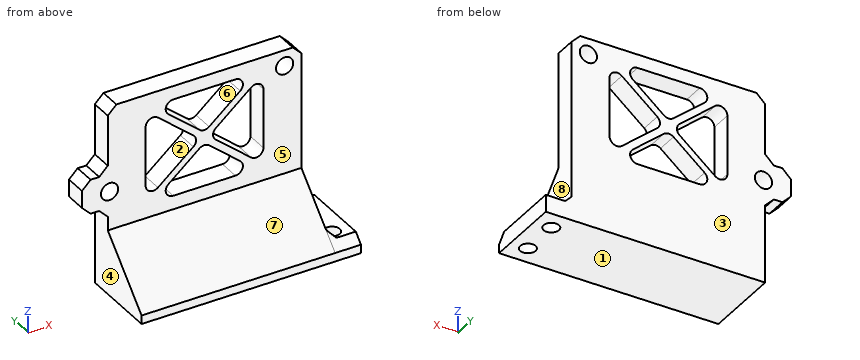
Autodesk Inventor part; units mm, degrees
ref_plane "作業平面2" through (-4, 15.3, 26.3) normal (0, -1, 0) x (1, 0, 0)
ref_plane "作業平面1" through (-4, 15.3, 26.3) normal (0, -1, 0) x (1, 0, 0)
ref_plane "作業平面3" through (45, 13, 3) normal (0, -1, 0) x (1, 0, 0)
sketch "スケッチ1" plane through (0, 0, 0) normal (0, 0, 1) x (1, 0, 0)
  line L0 (0, 0) -> (51, 0)
  line L1 (51, 0) -> (51, 18)
  line L2 (51, 18) -> (0, 18)
  line L3 (0, 18) -> (0, 0)
  circle A0 centre (47, 13.5) radius 1.8
  circle A1 centre (47, 4.5) radius 1.8
  dimension "d0" = 51
  dimension "d1" = 18
  dimension "d4" = 3.6
  dimension "d5" = 13.5
  dimension "d6" = 4
  dimension "d7" = 3.6
  dimension "d8" = 4
  dimension "d9" = 4.5
extrude "押し出し2" add sketch "スケッチ1" along normal blind 2
sketch "スケッチ2" plane through (0, 0, 2) normal (0, 0, 1) x (1, 0, 0)
  line L0 (0, 18) -> (0, 0)
  line L1 (0, 18) -> (44, 18)
  line L2 (44, 18) -> (44, 13)
  line L3 (44, 13) -> (0, 13)
  line L4 (0, 13) -> (0, 18)
  dimension "d12" = 44
  dimension "d13" = 5
extrude "押し出し3" add sketch "スケッチ2" along normal blind 42
sketch "スケッチ3" plane through (0, 13, 2) normal (0, -1, 0) x (1, 0, 0)
  circle A0 centre (41.1, 3.5) radius 2
  line L0 (44, 0) -> (44, 42)
  line L1 (44, 0) -> (0, 0)
  circle A1 centre (0.4, 19.8) radius 2
  point P0 (0, -2)
  dimension "d16" = 4
  dimension "d17" = 2.9
  dimension "d18" = 3.5
  dimension "d27" = 4
  dimension "d28" = 40.7
  dimension "d29" = 16.3
sketch "スケッチ4" plane through (0, 13, 2) normal (0, -1, 0) x (1, 0, 0)
  line L0 (8, 13.3) -> (-4, 13.3)
  line L1 (-4, 13.3) -> (-4, 24.3)
  line L2 (-4, 24.3) -> (8, 24.3)
  line L3 (8, 24.3) -> (8, 13.3)
  line L4 (44, 0) -> (0, 0)
  line L5 (44, 0) -> (44, 42)
  line L6 (0, 42) -> (44, 42)
  line L7 (0, 0) -> (0, 42)
  point P0 (0, -2)
  dimension "d19" = 13.3
  dimension "d20" = 36
  dimension "d25" = 11
  dimension "d26" = 12
ref_plane "作業平面2" through (-4, 15.3, 26.3) normal (0, -1, 0) x (1, 0, 0)
sketch "スケッチ5" plane through (-4, 15.3, 26.3) normal (0, -1, 0) x (1, 0, 0)
  point P0 (4, -26.3)
ref_plane "作業平面1" through (-4, 15.3, 26.3) normal (0, -1, 0) x (1, 0, 0)
sketch "スケッチ6" plane through (-4, 15.3, 26.3) normal (0, -1, 0) x (1, 0, 0)
  line L0 (4, -24.3) -> (4, 17.7)
  circle A0 centre (4.4, -2.3) radius 2
  circle A1 centre (45.1, 14) radius 2
  line L1 (4, -24.3) -> (55, -24.3)
  line L2 (48, -24.3) -> (48, 17.7)
  line L3 (4, 17.7) -> (48, 17.7)
  point P0 (4, -26.3)
  dimension "d45" = 4
  dimension "d46" = 0.4
  dimension "d47" = 4
  dimension "d48" = 22
  dimension "d49" = 2.9
  dimension "d67" = 43.8427
sketch "スケッチ7" plane through (0, 13, 2) normal (0, -1, 0) x (1, 0, 0)
  point P0 (0, -2)
sketch "スケッチ8" plane through (0, 13, 2) normal (0, -1, 0) x (1, 0, 0)
  line L0 (44, 0) -> (44, 42)
  line L1 (44, 0) -> (45, 0)
  line L2 (45, 0) -> (45, 21.3)
  line L3 (45, 21.3) -> (44, 21.3)
  line L4 (44, 21.3) -> (44, 0)
  point P0 (0, -2)
  dimension "d35" = 1
extrude "押し出し6" add sketch "スケッチ8" against normal blind 5
ref_plane "作業平面3" through (45, 13, 3) normal (0, -1, 0) x (1, 0, 0)
sketch "スケッチ9" plane through (45, 13, 3) normal (0, -1, 0) x (1, 0, 0)
  line L0 (-51, 17.2309) -> (-43, 17.2309)
  line L1 (-43, 17.2309) -> (-43, 25.2309)
  line L2 (-43, 25.2309) -> (-51, 25.2309)
  line L3 (-51, 25.2309) -> (-51, 17.2309)
  line L4 (0, 41) -> (-10, 41)
  line L5 (-10, 41) -> (-10, 7.258)
  line L6 (-10, 7.258) -> (0, 7.258)
  line L7 (0, 7.258) -> (0, 41)
  line L8 (0, 16.7) -> (0, 41)
  line L9 (-45, -1) -> (6, -1)
  point P0 (-45, -3)
  point P1 (-45, 4.4596)
  point P2 (-2.5771, 20.3)
  dimension "d55" = 8
  dimension "d59" = 0
  dimension "d97" = 18.2309
  dimension "d98" = 8.258
  dimension "d99" = 33.742
extrude "押し出し8" add sketch "スケッチ9" against normal blind 5
extrude "押し出し9" cut sketch "スケッチ6" along normal mid plane 10 contours A0 L0 | L0 A0 | A1
chamfer "面取り5" distance 13 angle 45 1 edges at (22.5, 13, 2)
sketch "スケッチ10" plane through (0, 0, 2) normal (0, 0, 1) x (1, 0, 0)
  line L0 (45, 18) -> (45, 0)
  line L1 (45, 0) -> (51, 0)
  line L2 (51, 0) -> (51, 18)
  line L3 (51, 18) -> (45, 18)
  circle A0 centre (47, 13.5) radius 1.8
  circle A1 centre (47, 4.5) radius 1.8
  circle A2 centre (47, 4.5) radius 1.8
  circle A3 centre (47, 13.5) radius 1.8
  line L4 (45, 0) -> (51, 0)
  line L5 (51, 0) -> (51, 18)
  line L6 (51, 18) -> (45, 18)
  line L7 (45, 18) -> (45, 0)
  point P0 (0, 0)
extrude "押し出し10" add sketch "スケッチ10" along normal blind 2
chamfer "面取り6" distance 2 angle 45 1 edges at (48, 0, 4)
chamfer "面取り7" distance 1.5 angle 45 1 edges at (45, 10.0001, 4)
chamfer "面取り8" distance 2 angle 45 4 edges at (45, 15.5, 44) (0, 15.5, 44) (-6, 15.5, 20.2309) (-6, 15.5, 28.2309)
sketch "スケッチ11" plane through (0, 13, 15) normal (0, -1, 0) x (1, 0, 0)
  line L0 (45, 0) -> (45, 27)
  line L1 (45, 13.5) -> (35.6998, 13.5)
  line L2 (19.8872, 15.8543) -> (11.6558, 22.7612)
  line L3 (21.4786, 14.5189) -> (32.2238, 14.5189) construction
  line L4 (19.8872, 13.1836) -> (11.6558, 6.2766)
  line L5 (21.4786, 14.5189) -> (32.2239, 14.5189) construction
  line L6 (8.7921, 7.612) -> (8.7921, 21.4259)
  arc A0 (11.6558, 22.7612) -> (8.7921, 21.4259) centre (10.5353, 21.4258) ccw
  arc A1 (19.8872, 13.1836) -> (19.8872, 15.8543) centre (18.7667, 14.5189) ccw
  arc A2 (8.7921, 7.612) -> (11.6558, 6.2766) centre (10.5353, 7.612) ccw
  line L7 (25.0769, 15.8544) -> (33.3082, 22.7613)
  line L8 (25.0769, 13.1835) -> (33.3082, 6.2766)
  line L9 (36.1721, 7.612) -> (36.1721, 21.4258)
  arc A3 (36.1721, 21.4258) -> (33.3082, 22.7613) centre (34.4288, 21.4258) ccw
  arc A4 (25.0769, 15.8544) -> (25.0769, 13.1835) centre (26.1975, 14.5189) ccw
  arc A5 (33.3082, 6.2766) -> (36.1721, 7.612) centre (34.4288, 7.612) ccw
  line L10 (23.55, 16.7078) -> (30.7794, 22.774)
  line L11 (23.8988, 16.5352) -> (33.3361, 16.5352) construction
  line L12 (21.3092, 16.7078) -> (14.0798, 22.774)
  line L13 (23.8988, 16.5352) -> (33.3361, 16.5352) construction
  line L14 (15.2002, 25.8522) -> (29.659, 25.8522)
  arc A6 (21.3092, 16.7078) -> (23.55, 16.7078) centre (22.4296, 18.043) ccw
  arc A7 (15.2002, 25.8522) -> (14.0798, 22.774) centre (15.2002, 24.1092) ccw
  arc A8 (30.7794, 22.774) -> (29.659, 25.8522) centre (29.659, 24.1092) ccw
  line L15 (23.5502, 12.3302) -> (30.7795, 6.2641)
  line L16 (21.309, 12.3302) -> (14.0797, 6.2641)
  line L17 (15.2003, 3.1853) -> (29.6589, 3.1853)
  arc A9 (23.5502, 12.3302) -> (21.309, 12.3302) centre (22.4296, 10.9947) ccw
  arc A10 (14.0797, 6.2641) -> (15.2003, 3.1853) centre (15.2003, 4.9286) ccw
  arc A11 (29.6589, 3.1853) -> (30.7795, 6.2641) centre (29.6589, 4.9286) ccw
  point P0 (0, -15)
  point P1 (8.7921, 25.1641)
  point P2 (8.792, 3.8737)
  point P3 (23.4854, 14.5189)
  point P4 (36.1721, 25.1643)
  point P5 (36.1721, 3.8735)
  point P6 (35.918, 26.6205)
  point P7 (11.8795, 26.6205)
  point P8 (21.9006, 14.5189)
  dimension "d82" = 16.561
  dimension "d83" = 140
  dimension "d84" = 16.5611
  dimension "d85" = 140
  dimension "d86" = 1.7432
  dimension "d87" = 15.69
  dimension "d88" = 40
  dimension "d89" = 15.69
  dimension "d90" = 140
  dimension "d91" = 1.743
extrude "押し出し11" cut sketch "スケッチ11" against normal blind 5
chamfer "面取り9" distance 2 angle 45 2 edges at (0, 15.5, 28.2309) (0, 15.5, 20.2309)
properties part number "PingCover-y" material "ABS プラスチック"
Geometry: final body of the model. Coordinates: model frame, mm. Face numbers are marked on the shaded views. A direction names the side the tool comes from. Round coordinates to 2 decimals unless told otherwise and drop trailing zeros. Write each loop counter-clockwise with the first axis right and the second up, starting at its lowest first coordinate (ties: lowest second). Pieces come first, ordered by that corner, then holes. Notation, with made-up numbers: (75, 51) -> (116, 51) arc R16 cw to (116, 77) -> close; hole circle Ø11 at (67.25, 66.5). An arc over 180 degrees is marked (long way). Return JSON: item names as keys, results as strings.
Q1. Mould query, pull axis X, two halves, no side actions, for the marked faces 6, 7 and 8. Classes: +X half, -X half, draft (parallel to the pull), parting line (faces both ways), or undercut.
From the geometry:
{"face 6": "undercut", "face 7": "draft", "face 8": "+X half"}
Q2. Section B-B on y = 4.5. Return the cut outline in (x, z), and give its area (3 significant figures).
From the geometry:
{"outline": "(0, 0) -> (45.2, 0) -> (45.2, 5.3) -> (45, 5.5) -> (45, 6.5) -> (0, 6.5) -> close; (48.8, 0) -> (51, 0) -> (51, 4) -> (48.8, 4) -> close", "area": "302 mm2"}
Q3. Ray query, line 1 (Y direction, x = 47, z = 1); line 2 (Y direction, x = 47, z = 3); line 3 (X direction, y = 16.4, z = 40.3). Return the intervals inside material, ascending.
From the geometry:
{"line 1": "0 to 2.7, 6.3 to 11.7, 15.3 to 18", "line 2": "1 to 2.7, 6.3 to 11.7, 15.3 to 18", "line 3": "0 to 13.93, 30.93 to 39.1, 43.1 to 45"}
Q4. First-contact query: pin 1 Ø1 at (y, z) = (9.5, 9) entering from -X; pin 2 Ø4 at (y, z) = (14.5, 28.5) entering from -X; pin 3 Ø3.5 at (x, y) = (49.5, 7.5) entering from +Z; pin 4 Ø10 at (y, z) = (12.5, 17.5) entering from -X. Flat tips, straight axial feed; report the tip coordinate or a pass-through.
From the geometry:
{"pin 1": "x = 0", "pin 2": "x = -5.73", "pin 3": "z = 4", "pin 4": "x = -6"}
Q5. Set-up query: the marked faces 1, 2, 3, 4 and 5. Return all of +Z, -Z, +X, -X, +Y, -Y with unobstructed straight access to the full face (end or side cutting, diameter ignored); none if empty.
From the geometry:
{"face 1": "-Z, +X, -X, +Y, -Y", "face 2": "+Y, -Y", "face 3": "+Z, -Z, +X, -X, +Y", "face 4": "-Z, -X, +Y, -Y", "face 5": "+Z, +X, -X, -Y"}
Q6. Section C-C on z = 39. Return the cut outline in (x, y).
From the geometry:
{"outline": "(0, 13) -> (13.46, 13) -> (13.46, 18) -> (0, 18) -> close; (31.4, 13) -> (39.58, 13) -> (39.58, 18) -> (31.4, 18) -> close; (42.62, 13) -> (45, 13) -> (45, 18) -> (42.62, 18) -> close"}
